from build123d import *

# Parameters (mm, degrees)
SKETCH_1_R      = 2
SKETCH_1_R_2    = 1.1
SKETCH_1_R_3    = 5.1
EXTRUDE_1_DEPTH = 2
FILLET_1_R      = 20


with BuildPart() as part:
    # ｽｹｯﾁ1 → ﾎﾞｽ - 押し出し1 (new body)
    with BuildSketch(Plane(origin=(0, 0, 0), x_dir=(1, 0, 0), z_dir=(0, 1, 0))):
        with BuildLine():
            ThreePointArc((-51.098969856, 31.700084423), (-56.508646061, 30.046179796), (-54.854741914, 24.636503444))
            Line((-54.854741914, 24.636503444), (-14.642511526, 3.255281279))
            ThreePointArc((-14.642511526, 3.255281279), (-12.857509511, -7.725571124), (-4, -14.456832295))
            Line((-4, -14.456832295), (-4, -60))
            ThreePointArc((-4, -60), (0, -64), (4, -60))
            Line((4, -60), (4, -14.456832295))
            ThreePointArc((4, -14.456832295), (12.857509511, -7.725571124), (14.642511526, 3.255281279))
            Line((14.642511526, 3.255281279), (54.854741789, 24.636503378))
            ThreePointArc((54.854741789, 24.636503378), (56.508645811, 30.046180267), (51.098968789, 31.700083856))
            Line((51.098968789, 31.700083856), (10.886739024, 10.318862022))
            ThreePointArc((10.886739024, 10.318862022), (0, 15), (-10.886739024, 10.318862022))
            Line((-10.886739024, 10.318862022), (-51.098969856, 31.700084423))
        make_face()
        with Locations(Location((0, -60, 0), (0, 0, 270))):
            Circle(SKETCH_1_R, mode=Mode.SUBTRACT)
        with Locations(Location((0, -37.5, 0), (0, 0, 270))):
            Circle(SKETCH_1_R, mode=Mode.SUBTRACT)
        with Locations(Location((-52.976855572, 28.168293767, 0), (0, 0, 270))):
            Circle(SKETCH_1_R, mode=Mode.SUBTRACT)
        with Locations(Location((-8.5, 0, 0), (0, 0, 270))):
            Circle(SKETCH_1_R_2, mode=Mode.SUBTRACT)
        with Locations(Location((0, 0, 0), (0, 0, 270))):
            Circle(SKETCH_1_R_3, mode=Mode.SUBTRACT)
        with Locations(Location((8.5, 0, 0), (0, 0, 270))):
            Circle(SKETCH_1_R_2, mode=Mode.SUBTRACT)
        with Locations(Location((52.976855572, 28.168293767, 0), (0, 0, 270))):
            Circle(SKETCH_1_R, mode=Mode.SUBTRACT)
    extrude(amount=EXTRUDE_1_DEPTH)

    # ﾌｨﾚｯﾄ1
    fillet_1_edges = [part.edges().sort_by_distance(p)[0] for p in [
        (-4, 1, 14.456832295),
        (-14.642511526, 1, -3.255281279),
        (-10.886739024, 1, -10.318862022),
        (10.886739024, 1, -10.318862022),
        (14.642511526, 1, -3.255281279),
        (4, 1, 14.456832295),
    ]]
    fillet(fillet_1_edges, radius=FILLET_1_R)


solid = part.part
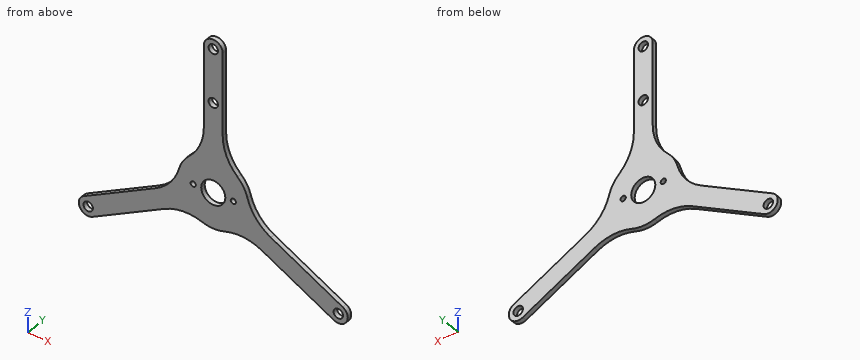
Check sheet for the modelled part. Datum: model origin and axes. Units: mm. Round coordinates to 2 decimals unless told otherwise and drop trailing zeros. Order: outer loops, then holes, each group sorted by start corner. A loop starts at its lowest first (then second) coordinate and runs counter-clockwise, first axis right, second up.
(1) Go/stop test with flat-tipped pins: P1, Ø0.6, axis at y = 1.5, z = 46.5, coming from the -X side; P2, Ø3, axis at x = 0, z = 37.5, coming from the -Y side; P3, Ø1, axis at y = 1, z = 41.5, coming from the +X side. Record where each tip stops, or that it passes through.
(2) Cross-section at A-A, the plane z = 37.5. Enter the section's corners in (x, y).
(3) Cross-section at B-B, the plane x = 0. Enter the section's corners in (y, z), and give its area (3 significant figures).
(4) Scan lines: probe 1 along X at (y, z) = (1.5, 0); probe 2 along X at (y, z) = (1.2, 37.5); probe 3 along X at (y, z) = (1.7, 28). Record each from-to range of solid material in increasing order.
(5) Cross-section at D-D, the plane z = -17.5. Enter the section's corners in (x, y), and give its area (3 significant figures).
(6) Cross-section at C-C, the plane y = 1.7. Enter the section's corners in (x, z).
Check sheet entries:
1. P1: stops at x = -4
1. P2: passes through
1. P3: stops at x = 4
2. outline: (-4, 0) - (-2, 0) - (-2, 2) - (-4, 2) - close; (2, 0) - (4, 0) - (4, 2) - (2, 2) - close
3. outline: (0, -15) - (2, -15) - (2, -5.1) - (0, -5.1) - close; (0, 5.1) - (2, 5.1) - (2, 35.5) - (0, 35.5) - close; (0, 39.5) - (2, 39.5) - (2, 58) - (0, 58) - close; (0, 62) - (2, 62) - (2, 64) - (0, 64) - close
3. area: 122 mm2
4. probe 1: x = -16.02 to -9.6, -7.4 to -5.1, 5.1 to 7.4, 9.6 to 16.02
4. probe 2: x = -4 to -2, 2 to 4
4. probe 3: x = -4 to 4
5. outline: (-41.43, 0) - (-24.39, 0) - (-24.39, 2) - (-41.43, 2) - close; (24.39, 0) - (41.43, 0) - (41.43, 2) - (24.39, 2) - close
5. area: 68.2 mm2
6. outline: (-54.85, -24.64) arc R4 ccw to (-51.1, -31.7) - (-20.62, -15.49) arc R20 cw to (-4.81, -14.21) arc R15 ccw to (4.81, -14.21) arc R20 cw to (20.62, -15.49) - (51.1, -31.7) arc R4 ccw to (54.85, -24.64) - (24.37, -8.43) arc R20 cw to (14.47, 3.96) arc R15 ccw to (10.29, 10.92) arc R20 cw to (4, 25.48) - (4, 60) arc R4 ccw to (-4, 60) - (-4, 25.48) arc R20 cw to (-10.29, 10.92) arc R15 ccw to (-14.47, 3.96) arc R20 cw to (-24.37, -8.43) - close; hole circle Ø4 at (-52.98, -28.17); hole circle Ø2.2 at (-8.5, 0); hole circle Ø10.2 at (0, 0); hole circle Ø4 at (0, 37.5); hole circle Ø4 at (0, 60); hole circle Ø2.2 at (8.5, 0); hole circle Ø4 at (52.98, -28.17)
